from build123d import *

# Parameters (mm, degrees)
SALIENTE_EXTRUIR1_DEPTH      = 2
CROQUIS2_W                   = 2.5
CROQUIS2_H                   = 4
SALIENTE_EXTRUIR2_DEPTH      = 5
SALIENTE_EXTRUIR3_DEPTH      = 2
SALIENTE_EXTRUIR3_DEPTH_BACK = 1


with BuildPart() as part:
    # Croquis1 → Saliente-Extruir1 (new body)
    with BuildSketch(Plane.XY):
        Polygon((44.714751496, -7.621064437), (44.114751496, -7.621064437), (44.114751496, -5.821064437), (45.220609876, -5.821064437), (45.220609876, -4.641064437), (45.220609876, -2.641064437), (43.114751496, -2.641064437), (43.114751496, -9.621064437), (44.114751496, -9.621064437), (45.220609876, -9.621064437), (45.220609876, -7.621064437), align=None)
    extrude(amount=SALIENTE_EXTRUIR1_DEPTH)

    # Croquis2 → Saliente-Extruir2 (add)
    with BuildSketch(Plane.XY.offset(2)):
        with Locations((43.970609876, -6.721064437)):
            Rectangle(CROQUIS2_W, CROQUIS2_H)
    extrude(amount=SALIENTE_EXTRUIR2_DEPTH)

    # Croquis3 → Saliente-Extruir3 (add, two sides: drawn at the far end of the back side and taken through both)
    with BuildSketch(Plane(origin=(0, 0, 0), x_dir=(-1, 0, 0), z_dir=(0, 0, -1)).offset(-SALIENTE_EXTRUIR3_DEPTH_BACK)):
        Polygon((-44.014751496, -2.37771269), (-44.014751496, -9.420966811), (-44.014751496, -11.420966811), (-45.220609876, -11.420966811), (-45.220609876, -13.420966811), (-40.220609876, -13.420966811), (-40.220609876, -12.420966811), (-40.220609876, 0.62228731), (-45.220609876, 0.62228731), (-45.220609876, -2.37771269), align=None)
    extrude(amount=SALIENTE_EXTRUIR3_DEPTH + SALIENTE_EXTRUIR3_DEPTH_BACK)


solid = part.part
Verification items for the finished model (mm, model axes). A direction names the side the tool comes from. Coordinates: 2 decimals unless noted, no trailing zeros. Order: outer loops, then holes, each group sorted by start corner. A loop starts at its lowest first (then second) coordinate and runs counter-clockwise, first axis right, second up. Notation, with made-up numbers: M -10.5,86 L 9.5,86 A34 ccw 9.5,123 Z; hole C 59,43.5 d8. An arc over 180 degrees is marked long. One line per item, written item: value. Start each with the question number.
Item 1: Scan lines: probe 1 along Z at (x, y) = (42.9, -6.25); probe 2 along Y at (x, z) = (44.95, -0.25); probe 3 along X at (y, z) = (-8.5, 4.75). Record each from-to range of solid material in increasing order.
Item 2: Sectioned sample at C-C (z = 0.5). Enter the section's corners in (x, y).
Item 3: Access from +Z, -Z, +X, -X, +Y, -Y to the whole of each face (thin tool, end or side, straight path). Record for faces 1 (the flat face through (44.4, -9.621, 1.2)), 2 (the flat face through (44, -8.721, 4)), 3 (the flat face through (44, -4, 2)), 4 (the flat face through (44.115, -7, 1)).
Item 4: Sectioned sample at A-A (x = 44.65). Enter the section's corners in (y, z).
Item 5: Mould release check, pull along Y, two halves, no side actions. Record for faces 5 (the flat face through (43, 0.622, 0)), 6 (the flat face through (45.221, -12, 0)), 7 (the flat face through (45, -2.378, 0)): released by +Y, released by -Y, zero draft, split by the parting line, or undercut.
Item 6: Gauge pin test, flat ends, axial feed: pin 1 (1.2 mm diameter, centred on x = 44, z = 5, fed in from -Y); pin 2 (1.7 mm diameter, centred on x = 44, y = -3, fed in from +Z); pin 3 (1.2 mm diameter, centred on y = -7, z = 4, fed in from -X). Record the tip position at first contact, or that the pin passes through.
Item 7: Sectioned sample at B-B (y = -6.5). Enter the section's corners in (x, z), then the cut area to 3 significant figures.
Item 8: Sectioned sample at D-D (x = 41.55). Enter the section's corners in (y, z), then the cut area to 3 significant figures.
Conclusion:
1. probe 1: z = -2 to 1, 2 to 7
1. probe 2: y = -13.42 to -11.42, -2.38 to 0.62
1. probe 3: x = 42.72 to 45.22
2. outline: M 40.22,-13.42 L 45.22,-13.42 L 45.22,-11.42 L 44.01,-11.42 L 44.01,-9.62 L 45.22,-9.62 L 45.22,-7.62 L 44.11,-7.62 L 44.11,-5.82 L 45.22,-5.82 L 45.22,-2.64 L 44.01,-2.64 L 44.01,-2.38 L 45.22,-2.38 L 45.22,0.62 L 40.22,0.62 Z
3. face 1: +Z, +X
3. face 2: +Z, +X, -X, -Y
3. face 3: +Z, +X, -X, +Y
3. face 4: -Z, +X
4. outline: M -13.42,-2 L -11.42,-2 L -11.42,1 L -13.42,1 Z; M -9.62,0 L -7.62,0 L -7.62,2 L -5.82,2 L -5.82,0 L -2.64,0 L -2.64,2 L -4.72,2 L -4.72,7 L -8.72,7 L -8.72,2 L -9.62,2 Z; M -2.38,-2 L 0.62,-2 L 0.62,1 L -2.38,1 Z
5. face 5: released by +Y
5. face 6: zero draft
5. face 7: undercut
6. pin 1: stops at y = -8.72
6. pin 2: stops at z = 2
6. pin 3: stops at x = 42.72
7. outline: M 40.22,-2 L 44.01,-2 L 44.01,0 L 44.11,0 L 44.11,2 L 45.22,2 L 45.22,7 L 42.72,7 L 42.72,2 L 43.11,2 L 43.11,1 L 40.22,1 Z
7. area: 25.0 mm^2
8. outline: M -13.42,-2 L 0.62,-2 L 0.62,1 L -13.42,1 Z
8. area: 42.1 mm^2
